Build history of the part. All positions in model axes, mm. A direction names the side the tool comes from. Give positions to 0.01 mm unless a question says otherwise; leave off trailing zeros. Loops run counter-clockwise (first coordinate to the right, second up) from the corner with the lowest first, then second, coordinate; pieces in that order, holes last. Notation, with made-up numbers: M 50.25,-15.75 L 87.25,-15.75 A23 ccw 87.25,8.25 Z; hole C 89.5,-29 d7. An arc over 180 degrees is marked long. Answer as a JSON object with one key per item and string values. Group by question number.
1. Slice it at B-B (z = -2.5). List the corners of the cut face in (x, y).
2. 3-axis set-ups, long thin cutter, end or side, ignore diameter. For faces 1 (the face through (6.35, 0, -3)), 2 (the face through (7, -13, 0)), 3 (the face through (-6, 6, 3.302)): which of +Z, -Z, +X, -X, +Y, -Y reach the whole face in a straight line?
3. Drop flat-ended pins along their axis: pin 1 Ø4 at (x, z) = (-15, 1) entering from +Y; pin 2 Ø1.5 at (y, z) = (11, -7.5) entering from +X; pin 3 Ø6 at (y, z) = (-0.5, -4) entering from +X. Give the stop position or say it passes through.
4. Drill centre lines: line 1 along Y through (x, z) = (0, 2.15); line 2 along Z through (x, y) = (12.5, 15.5); line 3 along Y through (x, z) = (-4, -7). Where is each one in solid material? Low to high. Write a range as [from, to].
5. Mould opens along Y. For faces 4 (the face through (3.131, 5.525, -3.137)), 5 (the face through (3.64, -27.7, 1.63)), 6 (the face through (-7, 0, -9.398)) say: released by +Y, released by -Y, zero draft, split by the parting line, or undercut.
6. Slice it at D-D (x = 19.5). List the corners of the cut face in (y, z).
7. Slice it at C-C (x = -1). List the corners of the cut face in (y, z) (3 decimals).
8. Slice it at A-A (y = 0). List the corners of the cut face in (x, z), then the cut area to 3 significant figures.
from build123d import *

# Parameters (mm, degrees)
SKETCH1_R           = 27.94
SKETCH1_R_2         = 2.032
BOSS_EXTRUDE1_DEPTH = 3.302
SKETCH2_R           = 14.224
BOSS_EXTRUDE2_DEPTH = 9.398
CUT_EXTRUDE1_DEPTH  = 12.7


with BuildPart() as part:
    # Sketch1 → Boss-Extrude1 (new body)
    with BuildSketch(Plane.XY):
        with Locations(Location((0, 0, 0), (0, 0, 180))):
            Circle(SKETCH1_R)
        with Locations(Location((0, 23.876, 0), (0, 0, 180))):
            Circle(SKETCH1_R_2, mode=Mode.SUBTRACT)
        with Locations(Location((20.677222541, 11.938, 0), (0, 0, 180))):
            Circle(SKETCH1_R_2, mode=Mode.SUBTRACT)
        with Locations(Location((20.677222541, -11.938, 0), (0, 0, 180))):
            Circle(SKETCH1_R_2, mode=Mode.SUBTRACT)
        with Locations(Location((0, -23.876, 0), (0, 0, 180))):
            Circle(SKETCH1_R_2, mode=Mode.SUBTRACT)
        with Locations(Location((-20.677222541, -11.938, 0), (0, 0, 180))):
            Circle(SKETCH1_R_2, mode=Mode.SUBTRACT)
        with Locations(Location((-20.677222541, 11.938, 0), (0, 0, 180))):
            Circle(SKETCH1_R_2, mode=Mode.SUBTRACT)
    extrude(amount=BOSS_EXTRUDE1_DEPTH)

    # Sketch2 → Boss-Extrude2 (add)
    with BuildSketch(Plane(origin=(0, 0, 0), x_dir=(-1, 0, 0), z_dir=(0, 0, -1))):
        with Locations(Location((0, 0, 0), (0, 0, 180))):
            Circle(SKETCH2_R)
    extrude(amount=BOSS_EXTRUDE2_DEPTH)

    # Sketch3 → Cut-Extrude1 (cut)
    with BuildSketch(Plane(origin=(0, 0, -9.398), x_dir=(-1, 0, 0), z_dir=(0, 0, -1))):
        Polygon((0, 7.332348419), (-6.35, 3.666174209), (-6.35, -3.666174209), (0, -7.332348419), (6.35, -3.666174209), (6.35, 3.666174209), align=None)
    extrude(amount=-CUT_EXTRUDE1_DEPTH, mode=Mode.SUBTRACT)


solid = part.part
Established:
{
 "1": {"outline": "C 0,0 d28.45; hole M -6.35,-3.67 L 0,-7.33 L 6.35,-3.67 L 6.35,3.67 L 0,7.33 L -6.35,3.67 Z"},
 "2": {"face 1": "+Z, -Z", "face 2": "-Z", "face 3": "+Z, +X, -X, +Y, -Y"},
 "3": {"pin 1": "stops at y = 24.73", "pin 2": "stops at x = 9.86", "pin 3": "stops at x = 14.22"},
 "4": {"line 1": "y = [-27.94, -25.91], [-21.84, -7.33], [7.33, 21.84], [25.91, 27.94]", "line 2": "z = [0, 3.3]", "line 3": "y = [-13.65, -5.02], [5.02, 13.65]"},
 "5": {"face 4": "undercut", "face 5": "split by the parting line", "face 6": "zero draft"},
 "6": {"outline": "M -20.01,0 L -13.59,0 L -13.59,3.3 L -20.01,3.3 Z; M -10.28,0 L 10.28,0 L 10.28,3.3 L -10.28,3.3 Z; M 13.59,0 L 20.01,0 L 20.01,3.3 L 13.59,3.3 Z"},
 "7": {"outline": "M -27.922,0 L -25.645,0 L -25.645,3.302 L -27.922,3.302 Z; M -22.107,0 L -14.189,0 L -14.189,-9.398 L -6.755,-9.398 L -6.755,3.302 L -22.107,3.302 Z; M 6.755,-9.398 L 14.189,-9.398 L 14.189,0 L 22.107,0 L 22.107,3.302 L 6.755,3.302 Z; M 25.645,0 L 27.922,0 L 27.922,3.302 L 25.645,3.302 Z"},
 "8": {"outline": "M -27.94,0 L -14.22,0 L -14.22,-9.4 L -6.35,-9.4 L -6.35,3.3 L -27.94,3.3 Z; M 6.35,-9.4 L 14.22,-9.4 L 14.22,0 L 27.94,0 L 27.94,3.3 L 6.35,3.3 Z", "area": "291 mm^2"}
}
